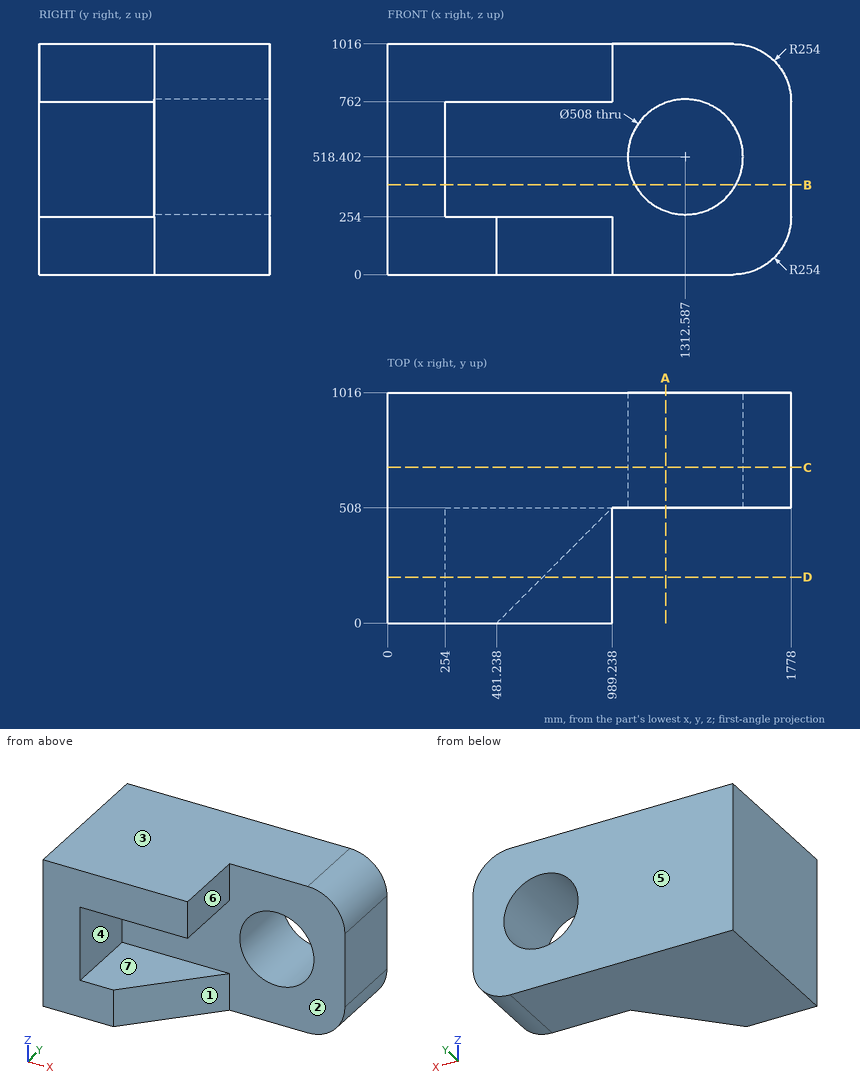
For this review, use the dimensioned drawing (mm, ordinates from the lowest corner) and the shaded views. A direction names the side the tool comes from. Coordinates: 2 decimals unless noted, no trailing zeros. Loops run counter-clockwise (first coordinate to the right, second up) from the corner with the lowest first, then second, coordinate; pieces in that order, holes last. Notation, with made-up numbers: (17, -5.75) -> (70, -5.75) arc R12 cw to (70, 15.25) -> close; hole circle Ø7 at (24, 11). An arc over 180 degrees is marked (long way). Use a Markdown table: item, result. Add a question column.
1. Add section A-A on x = 1226. Write out the cut boundary in (y, z).
2. Clearance check with flat-ended pins moving along their axes: pin 1 Ø3 at (x, z) = (671, 200.5) entering from -Y; pin 2 Ø5 at (y, z) = (233, 366) entering from +X; pin 3 Ø4 at (x, y) = (742, 163) entering from -Z. State where each tip first meets the part, or that it passes through.
3. Add section C-C on y = 686.5. Write out the cut boundary in (x, z), plus the area to 3 significant figures.
4. Add section D-D on y = 202.5. Write out the cut boundary in (x, z).
5. Draft analysis for pull direction Z (two halves, no side actions). For the marked faces 1, 2, 3 and 4, state which applies: pulls with the +Z half, pulls with the -Z half, needs draft (parallel to the pull), parting line crosses it, or undercut.
6. Add section B-B on z = 395.5. Write out the cut boundary in (x, y), plus the area to 3 significant figures.
7. To check wall thickness, follow line 1 (X direction, y = 319, z = 910.5); line 2 (Z direction, x = 953.5, y = 498); line 3 (X direction, y = 855.5, z = 690.5) (1 decimal). State the ranges of each line that lie inside material, in increasing order.
8. Machinability: for the marked faces 5, 6 and 7, which of the approach directions +Z, -Z, +X, -X, +Y, -Y give a long, thin tool a straight path to every point of the face, cutting with its end or side? Answer none if there is none.
Returned:
| question | item | result |
|---|---|---|
| 1 | outline | (508, 0) -> (1016, 0) -> (1016, 279.62) -> (508, 279.62) -> close; (508, 757.19) -> (1016, 757.19) -> (1016, 1016) -> (508, 1016) -> close |
| 2 | pin 1 | stops at y = 188.26 |
| 2 | pin 2 | stops at x = 254 |
| 2 | pin 3 | stops at z = 762 |
| 3 | outline | (0, 0) -> (1524, 0) arc R254 ccw to (1778, 254) -> (1778, 762) arc R254 ccw to (1524, 1016) -> (0, 1016) -> close; hole circle Ø508 at (1312.59, 518.4) |
| 3 | area | 1,580,000 mm² |
| 4 | outline | (0, 0) -> (683.74, 0) -> (683.74, 254) -> (254, 254) -> (254, 762) -> (989.24, 762) -> (989.24, 1016) -> (0, 1016) -> close |
| 5 | face 1 | needs draft |
| 5 | face 2 | undercut |
| 5 | face 3 | pulls with the +Z half |
| 5 | face 4 | undercut |
| 6 | outline | (0, 0) -> (254, 0) -> (254, 508) -> (1090.3, 508) -> (1090.3, 1016) -> (0, 1016) -> close; (1534.87, 508) -> (1778, 508) -> (1778, 1016) -> (1534.87, 1016) -> close |
| 6 | area | 806,000 mm² |
| 7 | line 1 | x = 0 to 989.24 |
| 7 | line 2 | z = 0 to 254, 762 to 1016 |
| 7 | line 3 | x = 0 to 1125.8, 1499.4 to 1778 |
| 8 | face 5 | +Z, -Z, +X, -X, +Y |
| 8 | face 6 | +Z, -Z, +X, -Y |
| 8 | face 7 | +X, -Y |
